```python
from build123d import *

# Parameters (mm, degrees)
EXTRUDE_THIN1_DEPTH = 10


with BuildPart() as part:
    # Sketch2 → Extrude-Thin1 (new, symmetric)
    with BuildSketch(Plane.XY):
        with BuildLine():
            Line((-161.781383655, 42.036480739), (-19.031512561, -35.182403693))
            ThreePointArc((-19.031512561, -35.182403693), (30.775705763, -25.551045669), (31.081700633, 25.177924573))
            Line((31.081700633, 25.177924573), (-46.806938551, 121.330066058))
            ThreePointArc((-46.806938551, 121.330066058), (-53.045839261, 126.247171893), (-60.793703836, 128))
            Line((-60.793703836, 128), (-221.819075448, 128))
            ThreePointArc((-221.819075448, 128), (-233.30903916, 123.855711237), (-239.508144262, 113.331192655))
            Line((-239.508144262, 113.331192655), (-260.223264765, 3.331192655))
            ThreePointArc((-260.223264765, 3.331192655), (-251.300991125, -15.720792041), (-230.403245845, -13.29812203))
            Line((-230.403245845, -13.29812203), (-170.979219548, 40.910276458))
            ThreePointArc((-170.979219548, 40.910276458), (-166.559963518, 42.940697498), (-161.781383655, 42.036480739))
        make_face()
        with BuildLine():
            Line((-159.402444585, 46.4342812), (-16.652573491, -30.784603232))
            ThreePointArc((-16.652573491, -30.784603232), (26.928742543, -22.35716496), (27.196488054, 22.030684001))
            Line((27.196488054, 22.030684001), (-50.69215113, 118.182825486))
            ThreePointArc((-50.69215113, 118.182825486), (-55.198023865, 121.734068589), (-60.793703836, 123))
            Line((-60.793703836, 123), (-221.819075448, 123))
            ThreePointArc((-221.819075448, 123), (-230.117382574, 120.00690256), (-234.594514036, 112.405861362))
            Line((-234.594514036, 112.405861362), (-255.309634539, 2.405861362))
            ThreePointArc((-255.309634539, 2.405861362), (-248.865770243, -11.353905363), (-233.772954208, -9.604199244))
            Line((-233.772954208, -9.604199244), (-174.348927911, 44.604199244))
            ThreePointArc((-174.348927911, 44.604199244), (-167.167636862, 47.903633434), (-159.402444585, 46.4342812))
        make_face(mode=Mode.SUBTRACT)
    extrude(amount=EXTRUDE_THIN1_DEPTH, both=True)


solid = part.part
```
The listing builds one solid part. Answer for the finished solid, in the listing's coordinates (mm). A direction names the side the tool comes from. Coordinates: 2 decimals unless noted, no trailing zeros. Loops run counter-clockwise (first coordinate to the right, second up) from the corner with the lowest first, then second, coordinate; pieces in that order, holes last. Notation, with made-up numbers: (37.25, 87) - (70.25, 87) arc R12 ccw to (70.25, 103) - close; hole circle Ø2 at (45, 62.5). An arc over 180 degrees is marked (long way). Use a Markdown table: item, result. Add a question column.
1) For faces 5 (the cylindrical face through (-233.17, 123.97, 0.14)), 6 (the flat face through (-140, 123, 0)), 7 (the flat face through (-91.41, 3.97, 0.14)), determine the directions among +Z, -Z, +X, -X, +Y, -Y from which every point of the face is accessible in a straight line to the end or side of a thin tool.
2) The part is cut by section B-B, the plane x = -211. Give the vertices of the cut face in (y, z).
3) The mould has two halves that part along X. Classify faces 1 (the flat face through (-140, 128, 0)), 2 (the flat face through (-249.72, 59.1, 0.14)), 3 (the flat face through (-244.807, 58.176, 0.14)), 4 (the cylindrical face through (-251.57, -15.57, 0.14)): released by +X, released by -X, zero draft, split by the parting line, or undercut.
4) Find the intervals of material crossed by line 1 (X direction, y = 27, z = -4.75); line 2 (Y direction, x = -8, z = 5); line 3 (X direction, y = 63.5, z = -1.75), in increasing order.
5) The part is cut by section A-A, the plane z = 5. Give the vertices of the cut face in (x, y), and give its area (3 significant figures).
6) The part is cut by section D-D, the plane y = -24.5. Give the vertices of the cut face in (x, z) (3 decimals).
7) The part is cut by section C-C, the plane y = 9.5. Give the vertices of the cut face in (x, z).
8) Given pin 1 (1.5 mm diameter, centred on y = 25, z = -7.5, fed in from +X); pin 2 (5 mm diameter, centred on y = 84, z = 1, fed in from +X); pin 3 (3 mm diameter, centred on y = 94, z = 6, fed in from +X), each flat-ended and moving along its own axis, determine where each tip first touches the part or whether it passes through.
Here are the results:
| question | item | result |
|---|---|---|
| 1 | face 5 | +Z, -Z, -X, +Y |
| 1 | face 6 | +Z, -Z |
| 1 | face 7 | +Z, -Z, -Y |
| 2 | outline | (4.4, -10) - (11.17, -10) - (11.17, 10) - (4.4, 10) - close; (123, -10) - (128, -10) - (128, 10) - (123, 10) - close |
| 3 | face 1 | zero draft |
| 3 | face 2 | released by -X |
| 3 | face 3 | undercut |
| 3 | face 4 | undercut |
| 4 | line 1 | x = -255.77 to -250.68, -193.65 to -186.23, -133.98 to -123.48, 23.17 to 29.61 |
| 4 | line 2 | y = -39.19 to -34.07, 65.48 to 73.42 |
| 4 | line 3 | x = -248.89 to -243.8, -6.4 to 0.04 |
| 5 | outline | (-260.22, 3.33) arc R18 ccw to (-230.4, -13.3) - (-170.98, 40.91) arc R8 cw to (-161.78, 42.04) - (-19.03, -35.18) arc R40 ccw to (31.08, 25.18) - (-46.81, 121.33) arc R18 ccw to (-60.79, 128) - (-221.82, 128) arc R18 ccw to (-239.51, 113.33) - close; hole (-255.31, 2.41) arc R13 ccw to (-233.77, -9.6) - (-174.35, 44.6) arc R13 cw to (-159.4, 46.43) - (-16.65, -30.78) arc R35 ccw to (27.2, 22.03) - (-50.69, 118.18) arc R13 ccw to (-60.79, 123) - (-221.82, 123) arc R13 ccw to (-234.59, 112.41) - close |
| 5 | area | 4,150 mm^2 |
| 6 | outline | (-38.779, -10) - (-28.271, -10) - (-28.271, 10) - (-38.779, 10) - close; (24.995, -10) - (31.619, -10) - (31.619, 10) - (24.995, 10) - close |
| 7 | outline | (-259.06, -10) - (-253.97, -10) - (-253.97, 10) - (-259.06, 10) - close; (-212.83, -10) - (-205.41, -10) - (-205.41, 10) - (-212.83, 10) - close; (-101.63, -10) - (-91.12, -10) - (-91.12, 10) - (-101.63, 10) - close; (33.69, -10) - (38.86, -10) - (38.86, 10) - (33.69, 10) - close |
| 8 | pin 1 | stops at x = 31.81 |
| 8 | pin 2 | stops at x = -14.54 |
| 8 | pin 3 | stops at x = -23.45 |
